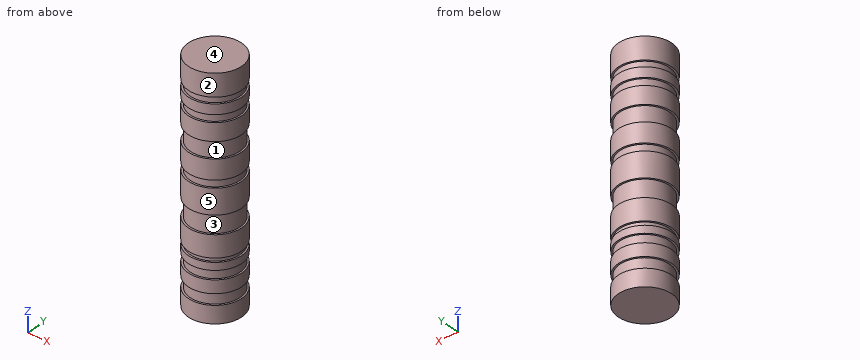
```python
from build123d import *

# Parameters (mm, degrees)
F0_R     = 11.4835992145
F0_R_2   = 10.7107701276
F1_DEPTH = 100
F2_W     = 32.8816715628
F2_H     = 2.6963576674
F2_W_2   = 32.8778307885
F2_H_2   = 3.1931251287
F2_W_3   = 32.5816031545
F2_H_3   = 6.9668218493
F2_W_4   = 32.9470410943
F2_H_4   = 3.193128854
F2_W_5   = 29.896620661
F2_H_5   = 7.8376792371
F2_H_6   = 1.7417054623
F2_W_6   = 27.0034540445
F2_H_7   = 3.7736967206
F2_W_7   = 26.4959204942
F2_H_8   = 4.6445494518
F4_DEPTH = 100


# Not quite as in the source:
# - a feature names something its author has since deleted; it is built from what else it names


with BuildPart() as f1:
    # F0 (on Top) → F1 (new body)
    with BuildSketch(Plane.XY):
        with Locations((-0.0411355359, -0.0693021866)):
            Circle(F0_R)
        Circle(F0_R_2, mode=Mode.SUBTRACT)
    extrude(amount=F1_DEPTH)

    # F2 (on Front) → F3 (revolve, cut)
    with BuildSketch(Plane.XZ):
        with Locations((-16.4408357814, 89.0894643962)):
            Rectangle(F2_W, F2_H)
        with Locations((-16.4389153942, 81.8779617548)):
            Rectangle(F2_W_2, F2_H_2)
        with Locations((-16.2908015773, 69.2505948246)):
            Rectangle(F2_W_3, F2_H_3)
        with Locations((-16.4735205472, 55.7523723692)):
            Rectangle(F2_W_4, F2_H_4)
        with Locations((-14.9483103305, 39.4964460284)):
            Rectangle(F2_W_5, F2_H_5)
        with Locations((-14.9483103305, 25.4176529124)):
            Rectangle(F2_W_5, F2_H_6)
        with Locations((-13.5017270222, 19.4668248296)):
            Rectangle(F2_W_6, F2_H_7)
        with Locations((-13.2479602471, 9.7422976978)):
            Rectangle(F2_W_7, F2_H_8)
    revolve(axis=Axis((0, 0, 49.8652271926), (0, 0, 1)), mode=Mode.SUBTRACT)

    # F0 (on Top) → F4 (join)
    with BuildSketch(Plane.XY):
        Circle(F0_R_2)
    extrude(amount=F4_DEPTH)


solid = f1.part
```
Could you check a few things on this model? Use its own coordinates, in mm. Face numbers are marked on the shaded views. A direction names the side the tool comes from. Round coordinates to 2 decimals unless told otherwise and drop trailing zeros. Loops run counter-clockwise (first coordinate to the right, second up) from the corner with the lowest first, then second, coordinate; pieces in that order, holes last.
Q1. I want a section at A-A (z = 59). Write out the boundary of the cut face in (x, y), and give its area (3 significant figures).
Q2. Please list where these lines run through material, in increasing order: L1, parallel to X at y = -0.5, z = 66; L2, parallel to Y at x = 3.25, z = 46; L3, parallel to X at y = 3.5, z = 74.
Q3. Thinking about a two-plate mould opening in Z: for the marked faces 3, 4 and 5, which applies, pulls with the +Z half, pulls with the -Z half, needs draft (parallel to the pull), parting line crosses it, or undercut?
Q4. On a 3-axis mill with a long thin cutter (end or side, diameter ignored), from which of +Z, -Z, +X, -X, +Y, -Y can I reach the whole of each face in a straight line? I mean the marked faces 1 and 2. Say none if no direction works.
Q5. For P1, Ø10, axis at y = -9, z = 23.5, coming from the -X side; P2, Ø1.5, axis at x = -2, z = 55.5, coming from the +Y side; P3, Ø1, axis at x = -8, z = 69, coming from the +Y side, each with a flat end and sliding along its axis, tell me the tip position at first contact or that it passes through.
Answer below:
1. outline: circle Ø22.97 at (-0.04, -0.07)
1. area: 414 mm2
2. L1: x = -10.7 to 10.7
2. L2: y = -11.07 to 10.93
2. L3: x = -10.96 to 10.87
3. face 3: undercut
3. face 4: pulls with the +Z half
3. face 5: needs draft
4. face 1: none
4. face 2: +Z, -Z
5. P1: stops at x = -10.83
5. P2: stops at y = 10.64
5. P3: stops at y = 7.65
